```python
from build123d import *

# Parameters (mm, degrees)
SKETCH_1_R      = 1.7
EXTRUDE_1_DEPTH = 3


with BuildPart() as part:
    # Эскиз1 → Бобышка-Вытянуть1 (new body)
    with BuildSketch(Plane(origin=(0, 0, 0), x_dir=(1, 0, 0), z_dir=(0, 1, 0))):
        with BuildLine():
            Line((-32.5, 3.5), (32.5, 3.5))
            ThreePointArc((32.5, 3.5), (36, 0), (32.5, -3.5))
            Line((32.5, -3.5), (-32.5, -3.5))
            ThreePointArc((-32.5, -3.5), (-36, 0), (-32.5, 3.5))
        make_face()
        Circle(SKETCH_1_R, mode=Mode.SUBTRACT)
        with BuildLine():
            Line((-32.5, -1.6), (-22.5, -1.6))
            ThreePointArc((-22.5, -1.6), (-20.9, 0), (-22.5, 1.6))
            Line((-22.5, 1.6), (-32.5, 1.6))
            ThreePointArc((-32.5, 1.6), (-34.1, 0), (-32.5, -1.6))
        make_face(mode=Mode.SUBTRACT)
        with BuildLine():
            Line((22.5, 1.6), (32.5, 1.6))
            ThreePointArc((32.5, 1.6), (34.1, 0), (32.5, -1.6))
            Line((32.5, -1.6), (22.5, -1.6))
            ThreePointArc((22.5, -1.6), (20.9, 0), (22.5, 1.6))
        make_face(mode=Mode.SUBTRACT)
    extrude(amount=EXTRUDE_1_DEPTH)


solid = part.part
```
Part model, mm, in its own coordinate system. A direction names the side the tool comes from. Round coordinates to 2 decimals unless told otherwise and drop trailing zeros. Loops run counter-clockwise (first coordinate to the right, second up) from the corner with the lowest first, then second, coordinate; pieces in that order, holes last. Notation, with made-up numbers: (-28, 28.5) -> (-18, 28.5) arc R34 ccw to (-18, 61.5) -> close; hole circle Ø6 at (24, -33.75). An arc over 180 degrees is marked (long way). Use a Markdown table: item, result.
1) Pull direction X, two halves, no side cores. Call faces 1 (the cylindrical face through (36, 1, 0)), 2 (the cylindrical face through (-34.1, 1.5, 0)), 3 (the flat face through (1, 3, -2)), 4 (the flat face through (27, 1, -1.6)): pulls with the +X half, pulls with the -X half, needs draft (parallel to the pull), parting line crosses it, or undercut.
The answers:
| item | result |
|---|---|
| face 1 | pulls with the +X half |
| face 2 | undercut |
| face 3 | needs draft |
| face 4 | undercut |
2) Cut at B-B, the plane z = 0. List the corners of the cut face in (x, y).
The answers:
| item | result |
|---|---|
| outline | (-36, 0) -> (-34.1, 0) -> (-34.1, 3) -> (-36, 3) -> close; (-20.9, 0) -> (-1.7, 0) -> (-1.7, 3) -> (-20.9, 3) -> close; (1.7, 0) -> (20.9, 0) -> (20.9, 3) -> (1.7, 3) -> close; (34.1, 0) -> (36, 0) -> (36, 3) -> (34.1, 3) -> close |
3) Cut at D-D, the plane x = 0. List the corners of the cut face in (y, z).
The answers:
| item | result |
|---|---|
| outline | (0, -3.5) -> (3, -3.5) -> (3, -1.7) -> (0, -1.7) -> close; (0, 1.7) -> (3, 1.7) -> (3, 3.5) -> (0, 3.5) -> close |
4) Cut at A-A, the plane x = -25.5. List the corners of the cut face in (y, z).
The answers:
| item | result |
|---|---|
| outline | (0, -3.5) -> (3, -3.5) -> (3, -1.6) -> (0, -1.6) -> close; (0, 1.6) -> (3, 1.6) -> (3, 3.5) -> (0, 3.5) -> close |
5) Tool access for faces 5 (the flat face through (1, 0, -2)), 6 (the cylindrical face through (20.9, 1.5, 0)): list every direction of +Z, -Z, +X, -X, +Y, -Y with a clear straight run to the whole face (end or side of a thin tool).
The answers:
| item | result |
|---|---|
| face 5 | +Z, -Z, +X, -X, -Y |
| face 6 | +Y, -Y |
6) Drop a flat-ended pin along its axis: pin 1 Ø4 at (x, z) = (0, 0) entering from -Y. Give the stop position or say it passes through.
The answers:
| item | result |
|---|---|
| pin 1 | stops at y = 0 |
7) Cut at C-C, the plane y = 0.7. List the corners of the cut face in (x, z), and give its area (3 significant figures).
The answers:
| item | result |
|---|---|
| outline | (-32.5, -3.5) -> (32.5, -3.5) arc R3.5 ccw to (32.5, 3.5) -> (-32.5, 3.5) arc R3.5 ccw to start; hole (-32.5, -1.6) -> (-22.5, -1.6) arc R1.6 ccw to (-22.5, 1.6) -> (-32.5, 1.6) arc R1.6 ccw to start; hole circle Ø3.4 at (0, 0); hole (22.5, -1.6) -> (32.5, -1.6) arc R1.6 ccw to (32.5, 1.6) -> (22.5, 1.6) arc R1.6 ccw to start |
| area | 404 mm2 |
8) Probe line 1 (X direction, y = 1, z = 0); line 2 (Z direction, x = 0, y = 1.5); line 3 (Z direction, x = 22.5, y = 0.55). List the from-to ranges inside material, lowest first. Write a range as [from, to].
The answers:
| item | result |
|---|---|
| line 1 | x = [-36, -34.1], [-20.9, -1.7], [1.7, 20.9], [34.1, 36] |
| line 2 | z = [-3.5, -1.7], [1.7, 3.5] |
| line 3 | z = [-3.5, -1.6], [1.6, 3.5] |
